```python
from build123d import *

# Parameters (mm, degrees)
BOSS_EXTRUDE1_DEPTH      = 1
BOSS_EXTRUDE1_DEPTH_BACK = 1.3622
SKETCH1_R                = 76.2
SKETCH1_R_2              = 1.6
SKETCH10_R               = 1.5
CUT_EXTRUDE4_DEPTH       = 108.788960422
SKETCH12_R               = 1.6
CUT_EXTRUDE6_DEPTH       = 108.788960422
SKETCH13_R               = 1.6
CUT_EXTRUDE7_DEPTH       = 10
SKETCH11_R               = 1.5
CUT_EXTRUDE5_DEPTH       = 10
SKETCH14_R               = 1.5875
SKETCH14_R_2             = 1.498962038
SKETCH14_W               = 10
SKETCH14_H               = 14
SKETCH14_W_2             = 41.679169521
SKETCH14_H_2             = 17.127679406
SKETCH14_W_3             = 21.415992251
SKETCH14_H_3             = 12
CUT_EXTRUDE8_DEPTH       = 10


with BuildPart() as part:
    # Sketch1 → Boss-Extrude1 (new, two sides: drawn at the far end of the back side and taken through both)
    with BuildSketch(Plane(origin=(0, 0, 0), x_dir=(1, 0, 0), z_dir=(0, 1, 0)).offset(-BOSS_EXTRUDE1_DEPTH_BACK)):
        with Locations(Location((0, 0, 0), (0, 0, 270))):
            Circle(SKETCH1_R)
        with Locations(Location((-41.747414599, 24.102881057, 0), (0, 0, 270))):
            Circle(SKETCH1_R_2, mode=Mode.SUBTRACT)
        with Locations(Location((41.747414599, 24.102881057, 0), (0, 0, 270))):
            Circle(SKETCH1_R_2, mode=Mode.SUBTRACT)
        with Locations(Location((0, -53.205762114, 0), (0, 0, 90))):
            Circle(SKETCH1_R_2, mode=Mode.SUBTRACT)
    extrude(amount=BOSS_EXTRUDE1_DEPTH + BOSS_EXTRUDE1_DEPTH_BACK)

    # Sketch10 → Cut-Extrude4 (cut, through all)
    with BuildSketch(Plane(origin=(0, 1, 0), x_dir=(1, 0, 0), z_dir=(0, 1, 0))):
        with Locations(Location((-5.6, -18, 0), (0, 0, 270))):
            Circle(SKETCH10_R)
        with Locations(Location((4, -18, 0), (0, 0, 90))):
            Circle(SKETCH10_R)
    extrude(amount=-CUT_EXTRUDE4_DEPTH, mode=Mode.SUBTRACT)

    # Sketch12 → Cut-Extrude6 (cut, through all)
    with BuildSketch(Plane(origin=(0, 1, 0), x_dir=(1, 0, 0), z_dir=(0, 1, 0))):
        with Locations(Location((-65.339987017, 24.618692946, 0), (0, 0, 270))):
            Circle(SKETCH12_R)
        with Locations(Location((-43.339987017, 30.618692946, 0), (0, 0, 270))):
            Circle(SKETCH12_R)
        with Locations(Location((-65.339987017, -29.381307054, 0), (0, 0, 270))):
            Circle(SKETCH12_R)
        with Locations(Location((-43.339987017, -29.381307054, 0), (0, 0, 270))):
            Circle(SKETCH12_R)
    extrude(amount=-CUT_EXTRUDE6_DEPTH, mode=Mode.SUBTRACT)

    # Sketch13 → Cut-Extrude7 (cut)
    with BuildSketch(Plane(origin=(0, 1, 0), x_dir=(1, 0, 0), z_dir=(0, 1, 0))):
        with Locations(Location((18.720998736, -45.143629297, 0), (0, 0, 270))):
            Circle(SKETCH13_R)
        with Locations(Location((52.719216113, 16.857348236, 0), (0, 0, 270))):
            Circle(SKETCH13_R)
        with Locations(Location((52.720998722, -45.142651738, 0), (0, 0, 270))):
            Circle(SKETCH13_R)
        with Locations(Location((18.719216128, 16.856370677, 0), (0, 0, 270))):
            Circle(SKETCH13_R)
    extrude(amount=-CUT_EXTRUDE7_DEPTH, mode=Mode.SUBTRACT)

    # Sketch11 → Cut-Extrude5 (cut)
    with BuildSketch(Plane(origin=(0, 1, 0), x_dir=(1, 0, 0), z_dir=(0, 1, 0))):
        with Locations(Location((36.103302507, 62.553143535, 0), (0, 0, 270))):
            Circle(SKETCH11_R)
        with Locations(Location((-29.973606883, 65.04314353, 0), (0, 0, 270))):
            Circle(SKETCH11_R)
        with Locations(Location((-29.973606883, 16.72314354, 0), (0, 0, 270))):
            Circle(SKETCH11_R)
    extrude(amount=-CUT_EXTRUDE5_DEPTH, mode=Mode.SUBTRACT)

    # Sketch14 → Cut-Extrude8 (cut)
    with BuildSketch(Plane(origin=(0, 1, 0), x_dir=(1, 0, 0), z_dir=(0, 1, 0))):
        with Locations(Location((-50.263897192, 50.100376278, 0), (0, 0, 270))):
            Circle(SKETCH14_R)
        with Locations(Location((-68.520147192, 18.479623722, 0), (0, 0, 270))):
            Circle(SKETCH14_R)
        with Locations(Location((18.25625, -68.58, 0), (0, 0, 270))):
            Circle(SKETCH14_R)
        with Locations(Location((-18.344787962, -68.58, 0), (0, 0, 270))):
            Circle(SKETCH14_R_2)
        with Locations(Location((50.263897192, 50.100376278, 0), (0, 0, 270))):
            Circle(SKETCH14_R)
        with Locations(Location((68.520147192, 18.479623722, 0), (0, 0, 270))):
            Circle(SKETCH14_R)
        with Locations(Location((-17.86667883, 16.903556997, 0), (0, 0, 270))):
            Circle(SKETCH14_R_2)
        with Locations((18.734359132, 16.903556997)):
            Circle(SKETCH14_R)
        with Locations(Location((-18.344787962, 68.58, 0), (0, 0, 270))):
            Circle(SKETCH14_R_2)
        with Locations(Location((18.25625, 68.58, 0), (0, 0, 270))):
            Circle(SKETCH14_R)
        with Locations(Location((-50.263897192, -50.100376278, 0), (0, 0, 270))):
            Circle(SKETCH14_R)
        with Locations(Location((-68.520147192, -18.479623722, 0), (0, 0, 270))):
            Circle(SKETCH14_R)
        with Locations(Location((50.263897192, -50.100376278, 0), (0, 0, 270))):
            Circle(SKETCH14_R)
        with Locations(Location((68.520147192, -18.479623722, 0), (0, 0, 270))):
            Circle(SKETCH14_R)
        with Locations((0, -70.602742007)):
            Rectangle(SKETCH14_W, SKETCH14_H)
        with Locations((9.16041524, 41.536536575)):
            Rectangle(SKETCH14_W_2, SKETCH14_H_2)
        with Locations((68.289586454, 0)):
            Rectangle(SKETCH14_W_3, SKETCH14_H_3)
    extrude(amount=-CUT_EXTRUDE8_DEPTH, mode=Mode.SUBTRACT)


solid = part.part
```
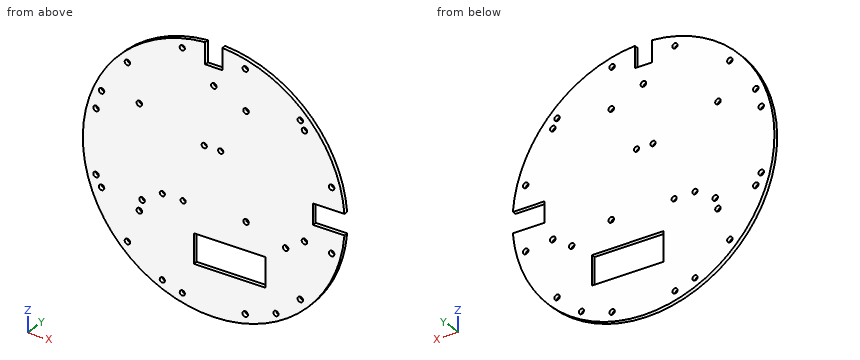
Geometry check sheet. Reference: the model listing, model coordinates, mm. Give positions to 0.01 mm unless a question says otherwise; leave off trailing zeros. Order: outer loops, then holes, each group sorted by start corner. A loop starts at its lowest first (then second) coordinate and runs counter-clockwise, first axis right, second up.
1. Section check A-A, the plane x = 7.5. Enter the section's corners in (y, z).
2. Section check C-C, the plane x = 32.5. Enter the section's corners in (y, z), and give its area (3 significant figures).
3. Section check B-B, the plane z = 0. Enter the section's corners in (x, y).
4. Gauge pin test, flat ends, axial feed: pin 1 Ø1.9 at (x, z) = (0, 53.21) entering from +Y; pin 2 Ø1 at (x, y) = (41.5, 0) entering from +Z. Record the tip position at first contact, or that the pin passes through.
5. Thickness scan on L1, parallel to Z at x = -43.5, y = 0.7; L2, parallel to Z at x = 17, y = -1.05; L3, parallel to X at y = -0.1, z = 18. Record the ranges inside material, lowest first.
6. Section check D-D, the plane y = -0.55. Give the number of separate pieces and of enclosed holes in the cut face, and give its area (3 significant figures).
Values follow:
1. outline: (-1.36, -75.83) - (1, -75.83) - (1, -50.1) - (-1.36, -50.1) - close; (-1.36, -32.97) - (1, -32.97) - (1, 75.83) - (-1.36, 75.83) - close
2. outline: (-1.36, -68.92) - (1, -68.92) - (1, 68.92) - (-1.36, 68.92) - close
2. area: 326 mm2
3. outline: (-76.2, -1.36) - (57.58, -1.36) - (57.58, 1) - (-76.2, 1) - close
4. pin 1: passes through
4. pin 2: stops at z = 64.23
5. L1: z = -62.56 to -32.21, -29.03 to 27.79, 30.97 to 62.56
5. L2: z = -74.28 to -69.55, -67.61 to -50.1, -32.97 to 67.61, 69.55 to 74.28
5. L3: x = -74.04 to -70.03, -67.01 to -7.1, -4.1 to 2.5, 5.5 to 67.01, 70.03 to 74.04
6. separate pieces: 1
6. enclosed holes: 30
6. area: 17,000 mm2
